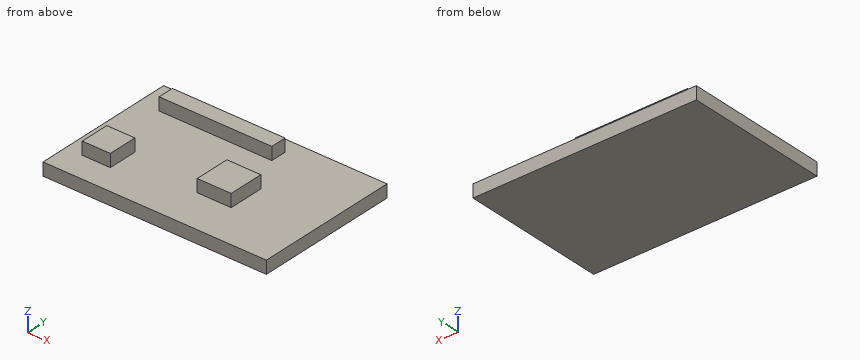
Autodesk Inventor part; units mm, degrees
ref_plane "YZ Plane" through (0, 0, 0) normal (1, 0, 0) x (0, 1, 0)
ref_plane "XZ Plane" through (0, 0, 0) normal (0, 1, 0) x (-1, 0, 0)
ref_plane "XY Plane" through (0, 0, 0) normal (0, 0, 1) x (1, 0, 0)
sketch "Sketch1" plane through (0, 0, 0) normal (0, 0, 1) x (1, 0, 0)
  line L0 (-5.4839, -45.5191) -> (-92.3615, -45.5191)
  line L1 (-92.3615, -45.5191) -> (-92.3615, 10.7724)
  line L2 (-92.3615, 10.7724) -> (-5.4839, 10.7724)
  line L3 (-5.4839, 10.7724) -> (-5.4839, -45.5191)
  point P0 (0, 0)
extrude "Extrusion1" add sketch "Sketch1" along normal blind 5
sketch "Sketch2" plane through (0, 0, 5) normal (0, 0, 1) x (1, 0, 0)
  point P0 (0, 0)
sketch "Sketch3" plane through (0, 0, 5) normal (0, 0, 1) x (1, 0, 0)
  line L0 (-40.3465, 5.0142) -> (-84.1809, 5.0142)
  line L1 (-84.1809, 5.0142) -> (-84.1809, -1.1473)
  line L2 (-84.1809, -1.1473) -> (-40.3465, -1.1473)
  line L3 (-40.3465, -1.1473) -> (-40.3465, 5.0142)
  line L4 (-74.8507, -23.6806) -> (-85.7653, -23.6806)
  line L5 (-85.7653, -23.6806) -> (-85.7653, -35.1234)
  line L6 (-85.7653, -35.1234) -> (-74.8507, -35.1234)
  line L7 (-74.8507, -35.1234) -> (-74.8507, -23.6806)
  line L8 (-32.6006, -15.5827) -> (-45.8038, -15.5827)
  line L9 (-45.8038, -15.5827) -> (-45.8038, -29.402)
  line L10 (-45.8038, -29.402) -> (-32.6006, -29.402)
  line L11 (-32.6006, -29.402) -> (-32.6006, -15.5827)
  point P0 (0, 0)
extrude "Extrusion2" add sketch "Sketch3" along normal blind 5
properties part number "raspberry"
Work out the finished part from the listing and answer in its coordinate system (mm). Give positions to 0.01 mm unless a question says otherwise; leave off trailing zeros. Order: outer loops, then holes, each group sorted by start corner. A loop starts at its lowest first (then second) coordinate and runs counter-clockwise, first axis right, second up. Notation, with made-up numbers: M 60,17 L 90,17 A9 ccw 90,30 Z; hole C -10,60 d10. An arc over 180 degrees is marked long. Return JSON: item names as keys, results as strings.
1) Straight lines are drawn through the part: line 1 along X through (y, z) = (-28, 5.75); line 2 along Z through (x, y) = (-18.5, -12); line 3 along X through (y, z) = (-30, 5.5). For each, find the intervals that lie inside material, in ascending order. Write a range as [from, to].
Resolved:
{"line 1": "[-85.77, -74.85], [-45.8, -32.6]", "line 2": "[0, 5]", "line 3": "[-85.77, -74.85]"}
2) Section C-C, the plane y = -25 is taken. Write down the section's boundary in (x, z), plus the area to 3 significant figures.
Resolved:
{"outline": "M -92.36,0 L -5.48,0 L -5.48,5 L -32.6,5 L -32.6,10 L -45.8,10 L -45.8,5 L -74.85,5 L -74.85,10 L -85.77,10 L -85.77,5 L -92.36,5 Z", "area": "555 mm^2"}
3) Section B-B, the plane x = -43.5 is taken. Write down the section's boundary in (y, z).
Resolved:
{"outline": "M -45.52,0 L 10.77,0 L 10.77,5 L 5.01,5 L 5.01,10 L -1.15,10 L -1.15,5 L -15.58,5 L -15.58,10 L -29.4,10 L -29.4,5 L -45.52,5 Z"}
4) Section A-A, the plane z = 6 is taken. Write down the section's boundary in (x, y), plus the area to 3 significant figures.
Resolved:
{"outline": "M -85.77,-35.12 L -74.85,-35.12 L -74.85,-23.68 L -85.77,-23.68 Z; M -84.18,-1.15 L -40.35,-1.15 L -40.35,5.01 L -84.18,5.01 Z; M -45.8,-29.4 L -32.6,-29.4 L -32.6,-15.58 L -45.8,-15.58 Z", "area": "577 mm^2"}
5) Section D-D, the plane y = 1 is taken. Write down the section's boundary in (x, z), plus the area to 3 significant figures.
Resolved:
{"outline": "M -92.36,0 L -5.48,0 L -5.48,5 L -40.35,5 L -40.35,10 L -84.18,10 L -84.18,5 L -92.36,5 Z", "area": "654 mm^2"}
6) Each of these flat-tipped pins is pushed along its axis until it touches: pin 1 (5.5 mm diameter, centred on y = -28, z = 8.5, fed in from -X); pin 2 (5.5 mm diameter, centred on x = -40.5, z = 6.5, fed in from +Y); pin 3 (4 mm diameter, centred on x = -42, z = 8.5, fed in from -Y); pin 4 (1 mm diameter, centred on x = -67, z = 7, fed in from +Y). Where does it stop, or does it pass through?
Resolved:
{"pin 1": "x = -85.77", "pin 2": "y = 10.77", "pin 3": "y = -29.4", "pin 4": "y = 5.01"}
